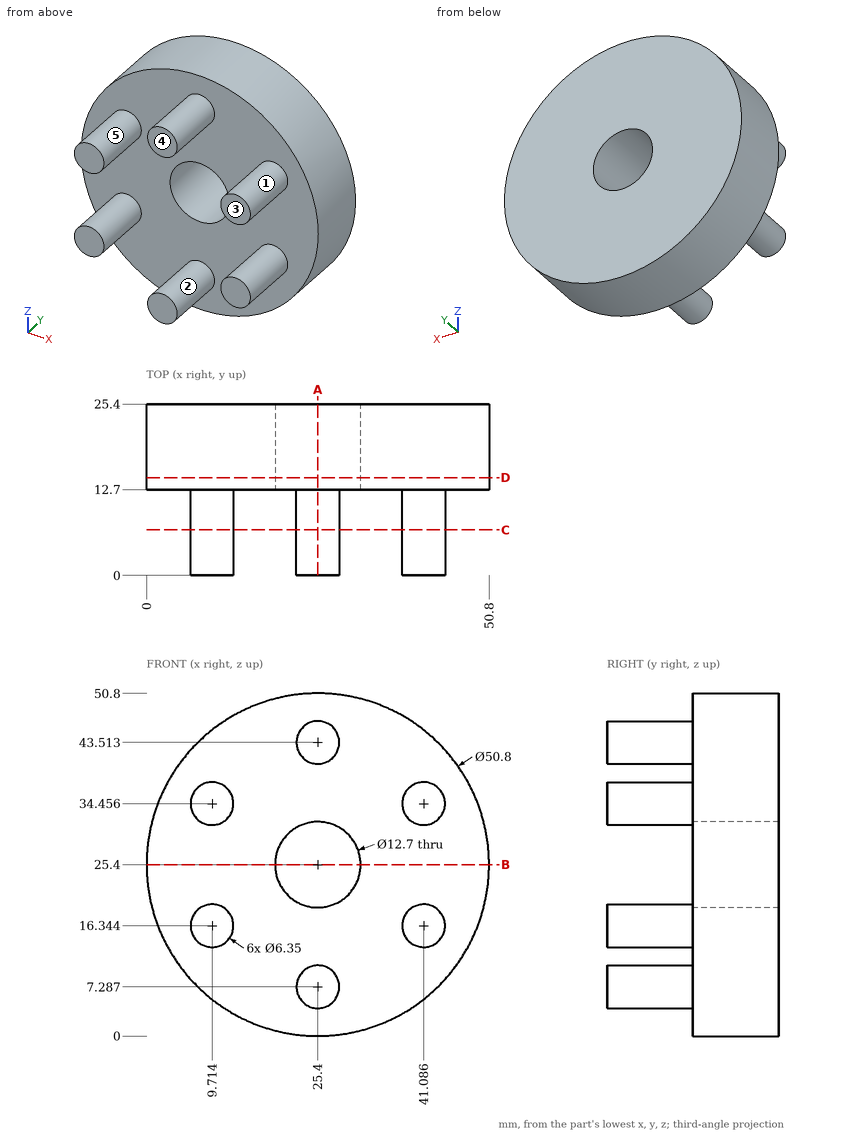
Answer from the drawing. Dimensions are ordinates in mm from the lowest x, y and z of the part. A direction names the side the tool comes from. Give positions to 0.01 mm unless a question says otherwise; leave off trailing zeros. Loops run counter-clockwise (first coordinate to the right, second up) from the corner with the lowest first, then second, coordinate; pieces in that order, holes last.
Item 1: The mould has two halves that part along X. Classify the marked faces 1, 2 and 3: released by +X, released by -X, zero draft, split by the parting line, or undercut.
Item 2: Each of these flat-tipped pins is pushed along its axis until it touches: pin 1 Ø10 at (x, z) = (16.5, 28.5) entering from -Y; pin 2 Ø1 at (x, y) = (11, 3.5) entering from -Z; pin 3 Ø3 at (y, z) = (6.5, 6) entering from -X (3 decimals). Where does it stop, or does it pass through?
Item 3: The part is cut by section C-C (y = 6.75). Give the number of separate pieces and of enclosed holes in the cut face, and give its area (3 significant figures).
Item 4: For the marked faces 4 and 5, determine the directions among +Z, -Z, +X, -X, +Y, -Y from which every point of the face is accessible in a straight line to the end or side of a thin tool.
Item 5: The part is cut by section B-B (z = 25.4). Write down the section's boundary in (x, y), and give its area (3 significant figures).
Item 6: The part is cut by section A-A (x = 25.4). Write down the section's boundary in (y, z).
Item 7: The part is cut by section D-D (y = 14.5). Write down the section's boundary in (x, z).
Item 8: Find the intervals of material crossed by line 1 along Z through (x, y) = (25.4, 19.25); line 2 along Y through (x, z) = (18.5, 34); line 3 along X through (y, z) = (6, 18) (1 decimal), in increasing order.
Taken from the geometry:
1. face 1: undercut
1. face 2: split by the parting line
1. face 3: zero draft
2. pin 1: stops at y = 12.7
2. pin 2: stops at z = 13.27
2. pin 3: stops at x = 22.225
3. separate pieces: 6
3. enclosed holes: 0
3. area: 190 mm2
4. face 4: +Z, -Z, +X, -X, -Y
4. face 5: -Y
5. outline: (0, 12.7) - (19.05, 12.7) - (19.05, 25.4) - (0, 25.4) - close; (31.75, 12.7) - (50.8, 12.7) - (50.8, 25.4) - (31.75, 25.4) - close
5. area: 484 mm2
6. outline: (0, 4.11) - (12.7, 4.11) - (12.7, 0) - (25.4, 0) - (25.4, 19.05) - (12.7, 19.05) - (12.7, 10.46) - (0, 10.46) - close; (0, 40.34) - (12.7, 40.34) - (12.7, 31.75) - (25.4, 31.75) - (25.4, 50.8) - (12.7, 50.8) - (12.7, 46.69) - (0, 46.69) - close
7. outline: circle Ø50.8 at (25.4, 25.4); hole circle Ø12.7 at (25.4, 25.4)
8. line 1: z = 0 to 19.05, 31.75 to 50.8
8. line 2: y = 12.7 to 25.4
8. line 3: x = 7 to 12.4, 38.4 to 43.8
